Input: part model. Units: mm. Frame: model coordinates. Coordinates: 2 decimals unless noted, no trailing zeros. Write each loop counter-clockwise with the first axis right and the second up, starting at its lowest first coordinate (ties: lowest second). Pieces come first, ordered by that corner, then holes. Notation, with made-up numbers: (-36.5, 6.5) - (-22.5, 6.5) arc R8 ccw to (-22.5, 10.5) - close; hole circle Ø4 at (34.25, -16.75). An arc over 180 degrees is marked (long way). Use CSV: the item, a comma, the result in double quotes.
```python
from build123d import *

# Parameters (mm, degrees)
CROQUIS1_R              = 6
SALIENTE_EXTRUIR1_DEPTH = 3.7


with BuildPart() as part:
    # Croquis1 → Saliente-Extruir1 (new body)
    with BuildSketch(Plane(origin=(0, 0, 0), x_dir=(1, 0, 0), z_dir=(0, 1, 0))):
        Polygon((0, 9.814954576), (-8.5, 4.907477288), (-8.5, -4.907477288), (0, -9.814954576), (8.5, -4.907477288), (8.5, 4.907477288), align=None)
        with Locations(Location((0, 0, 0), (0, 0, 270))):
            Circle(CROQUIS1_R, mode=Mode.SUBTRACT)
    extrude(amount=SALIENTE_EXTRUIR1_DEPTH)

    # Croquis2 → Cortar-Revolución1 (revolve, cut)
    with BuildSketch(Plane(origin=(0, 0, 0), x_dir=(0, 0, -1), z_dir=(1, 0, 0))):
        with BuildLine():
            Line((7.814954576, 3.7), (9.814954576, 3.7))
            Line((9.814954576, 3.7), (9.814954576, 3.05))
            ThreePointArc((9.814954576, 3.05), (8.866441618, 3.533421668), (7.814954576, 3.7))
        make_face()
        with BuildLine():
            Line((9.814954576, 0.65), (9.814954576, 0))
            Line((9.814954576, 0), (7.814954576, 0))
            ThreePointArc((7.814954576, 0), (8.866441618, 0.166578332), (9.814954576, 0.65))
        make_face()
    revolve(axis=Axis((0, 0, 0), (0, 1, 0)), mode=Mode.SUBTRACT)


solid = part.part
```
(1) Cut plane C-C on y = 3.35. Return loops of the section in (x, z).
Check values:
outline,"(-8.5, -3.82) arc R9.32 ccw to (-7.56, -5.45) - (-0.94, -9.27) arc R9.32 ccw to (0.94, -9.27) - (7.56, -5.45) arc R9.32 ccw to (8.5, -3.82) - (8.5, 3.82) arc R9.32 ccw to (7.56, 5.45) - (0.94, 9.27) arc R9.32 ccw to (-0.94, 9.27) - (-7.56, 5.45) arc R9.32 ccw to (-8.5, 3.82) - close; hole circle Ø12 at (0, 0)"
(2) Cut plane B-B on z = 0. Return loops of the section in (x, y), and give its area (3 significant figures).
Check values:
outline,"(-8.5, 0.07) arc R3.4 ccw to (-7.81, 0) - (-6, 0) - (-6, 3.7) - (-7.81, 3.7) arc R3.4 ccw to (-8.5, 3.63) - close; (6, 0) - (7.81, 0) arc R3.4 ccw to (8.5, 0.07) - (8.5, 3.63) arc R3.4 ccw to (7.81, 3.7) - (6, 3.7) - close"
area,"18.4 mm^2"
(3) Cut plane A-A on y = 1.1. Return loops of the section in (x, z), and give its area (3 significant figures).
Check values:
outline,"(-8.5, -4.91) - (0, -9.81) - (8.5, -4.91) - (8.5, 4.91) - (0, 9.81) - (-8.5, 4.91) - close; hole circle Ø12 at (0, 0)"
area,"137 mm^2"
(4) Draft query along X for faces 1 (the flat face through (-2, 3.7, 6)), 2 (the flat face through (8.5, 2, 0)), 3 (the cylindrical face through (1.802, 1.824, 5.723)). Return one class per face: pulls with the +X half, pulls with the -X half, needs draft (parallel to the pull), parting line crosses it, or undercut.
Check values:
face 1,"needs draft"
face 2,"pulls with the +X half"
face 3,"undercut"
(5) Ray query, probe 1 along X at (y, z) = (2.15, 0); probe 2 along Z at (x, y) = (-1, 2.15); probe 3 along X at (y, z) = (1.3, -2.75). Return the intervals inside material, ascending. Write a range as from..to.
Check values:
probe 1,"-8.5..-6, 6..8.5"
probe 2,"-9.24..-5.92, 5.92..9.24"
probe 3,"-8.5..-5.33, 5.33..8.5"
